Part print with two shaded views. Sizes in mm from the minimum x, y, z corner. A direction names the side the tool comes from. Give positions to 0.01 mm unless a question says otherwise; leave off trailing zeros. Order: outer loops, then holes, each group sorted by start corner. A loop starts at its lowest first (then second) coordinate and runs counter-clockwise, first axis right, second up. Notation, with made-up numbers: (24, 37) -> (39, 37) arc R20 ccw to (39, 44) -> close; hole circle Ø9 at (47.25, 77). An arc over 180 degrees is marked (long way). Write item = value, one per line. Start each with the question number.
Item 1: Flat gauge pins, fed straight in: P1, Ø2, axis at x = 11, y = 10.5, coming from the +Z side; P2, Ø2, axis at x = 10.5, z = 4, coming from the +Y side; P3, Ø1.5, axis at x = 5, z = 1.5, coming from the +Y side. Where does each tip first touch, or does it go through?
Item 2: Band-saw the part on A-A on x = 9. Write the cut outline in (y, z), plus the area to 3 significant figures.
Item 3: Drill centre lines: line 1 along Y through (x, z) = (9, 4.8); line 2 along Z through (x, y) = (7, 11.75); line 3 along Y through (x, z) = (9, 3.1). Where is each one in solid material? Low to high.
Item 4: Pull direction X, two halves, no side cores. Call the marked faces 3, 4 and 5: +X half, -X half, draft (parallel to the pull), parting line (faces both ways), or undercut.
Item 5: Band-saw the part on C-C on z = 6.5. Write the cut outline in (x, y).
Item 6: Band-saw the part on B-B on z = 7.75. Write the cut outline in (x, y), plus the area to 3 significant figures.
Item 7: Tool access for the marked faces 1 and 2: list every direction of +Z, -Z, +X, -X, +Y, -Y with a clear straight run to the whole face (end or side of a thin tool).
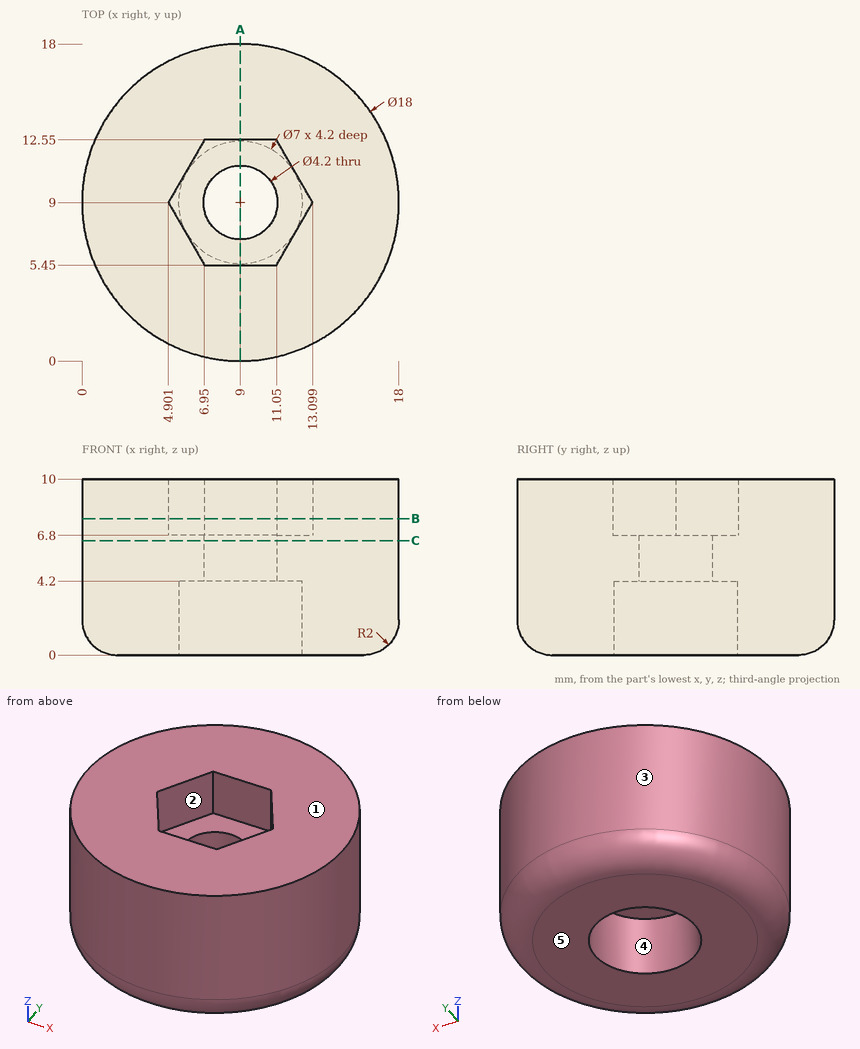
Values found:
q1.P1 = 6.8
q1.P2 = 17.99
q1.P3 = 17.36
q2.outline = (0, 2) arc R2 ccw to (2, 0) -> (5.5, 0) -> (5.5, 4.2) -> (6.9, 4.2) -> (6.9, 6.8) -> (5.45, 6.8) -> (5.45, 10) -> (0, 10) -> close; (11.1, 4.2) -> (12.5, 4.2) -> (12.5, 0) -> (16, 0) arc R2 ccw to (18, 2) -> (18, 10) -> (12.55, 10) -> (12.55, 6.8) -> (11.1, 6.8) -> close
q2.area = 115 mm^2
q3.line_1 = 0 to 6.9, 11.1 to 18
q3.line_2 = 4.2 to 6.8
q3.line_3 = 0 to 5.5, 12.5 to 18
q4.face_3 = parting line
q4.face_4 = undercut
q4.face_5 = draft
q5.outline = circle Ø18 at (9, 9); hole circle Ø4.2 at (9, 9)
q6.outline = circle Ø18 at (9, 9); hole (4.9, 9) -> (6.95, 5.45) -> (11.05, 5.45) -> (13.1, 9) -> (11.05, 12.55) -> (6.95, 12.55) -> close
q6.area = 211 mm^2
q7.face_1 = +Z, +X, -X, +Y, -Y
q7.face_2 = +Z
